Autodesk Inventor part; units mm, degrees
ref_plane "YZ Plane" through (0, 0, 0) normal (1, 0, 0) x (0, 1, 0)
ref_plane "XZ Plane" through (0, 0, 0) normal (0, 1, 0) x (-1, 0, 0)
ref_plane "XY Plane" through (0, 0, 0) normal (0, 0, 1) x (1, 0, 0)
sketch "Esquisse1" plane through (0, 0, 0) normal (0, 0, 1) x (1, 0, 0)
  circle A0 centre (0, 0) radius 13.75
  dimension "d0" = 27.5
extrude "Extrusion1" add sketch "Esquisse1" along normal blind 37.5
sketch "Esquisse2" plane through (0, 0, 0) normal (0, 0, -1) x (-1, 0, 0)
  circle A0 centre (0, 0) radius 5
  dimension "d3" = 10
extrude "Extrusion2" add sketch "Esquisse2" along normal blind 3.5
sketch "Esquisse3" plane through (0, 0, 37.5) normal (0, 0, 1) x (1, 0, 0)
  circle A0 centre (0, 0) radius 1.2
  dimension "d6" = 2.4
extrude "Extrusion3" add sketch "Esquisse3" along normal blind 13
sketch "Esquisse4" plane through (0, 0, 37.5) normal (0, 0, 1) x (1, 0, 0)
  circle A0 centre (0, 0) radius 1.2
  circle A1 centre (0, 0) radius 5
  dimension "d9" = 10
extrude "Extrusion4" add sketch "Esquisse4" along normal blind 3.5
fillet "Congé1" radius 1 2 edges at (-5, 0, 41) (5, 0, -3.5)
fillet "Congé2" radius 1 1 edges at (-13.75, 0, 37.5)
fillet "Congé3" radius 0.5 1 edges at (-1.2, 0, 50.5)
sketch "Esquisse5" plane through (0, 0, 37.5) normal (0, 0, 1) x (1, 0, 0)
  circle A0 centre (0, 8) radius 1
  arc A1 (7.7336, 4.6035) -> (4.9749, 7.5) centre (0, 0) ccw construction
  arc A2 (9.0225, 5.3707) -> (5.8041, 8.75) centre (0, 0) ccw
  arc A3 (6.4446, 3.8362) -> (4.1458, 6.25) centre (0, 0) ccw
  arc A4 (6.4446, 3.8362) -> (9.0225, 5.3707) centre (7.7336, 4.6035) ccw
  arc A5 (5.8041, 8.75) -> (4.1458, 6.25) centre (4.9749, 7.5) ccw
  line L0 (0, 0) -> (0, 21.7918) construction
  circle A6 centre (0, -8) radius 1
  arc A7 (8.75, -5.8041) -> (6.25, -4.1458) centre (7.5, -4.9749) ccw
  arc A8 (5.3707, -9.0225) -> (8.75, -5.8041) centre (0, 0) ccw
  arc A9 (3.8362, -6.4446) -> (5.3707, -9.0225) centre (4.6035, -7.7336) ccw
  arc A10 (3.8362, -6.4446) -> (6.25, -4.1458) centre (0, 0) ccw
  arc A11 (-5.8041, -8.75) -> (-4.1458, -6.25) centre (-4.9749, -7.5) ccw
  arc A12 (-9.0225, -5.3707) -> (-5.8041, -8.75) centre (0, 0) ccw
  arc A13 (-6.4446, -3.8362) -> (-9.0225, -5.3707) centre (-7.7336, -4.6035) ccw
  arc A14 (-6.4446, -3.8362) -> (-4.1458, -6.25) centre (0, 0) ccw
  arc A15 (-8.75, 5.8041) -> (-6.25, 4.1458) centre (-7.5, 4.9749) ccw
  arc A16 (-5.3707, 9.0225) -> (-8.75, 5.8041) centre (0, 0) ccw
  arc A17 (-3.8362, 6.4446) -> (-5.3707, 9.0225) centre (-4.6035, 7.7336) ccw
  arc A18 (-3.8362, 6.4446) -> (-6.25, 4.1458) centre (0, 0) ccw
  dimension "d15" = 2
  dimension "d16" = 3
  dimension "d17" = 8
  dimension "d19" = 7
  dimension "d21" = 5
  dimension "d22" = 9
  dimension "d25" = 360
  dimension "d29" = 360
extrude "Extrusion5" cut sketch "Esquisse5" against normal blind 5
properties part number "Moteur" material "Acier inoxydable"
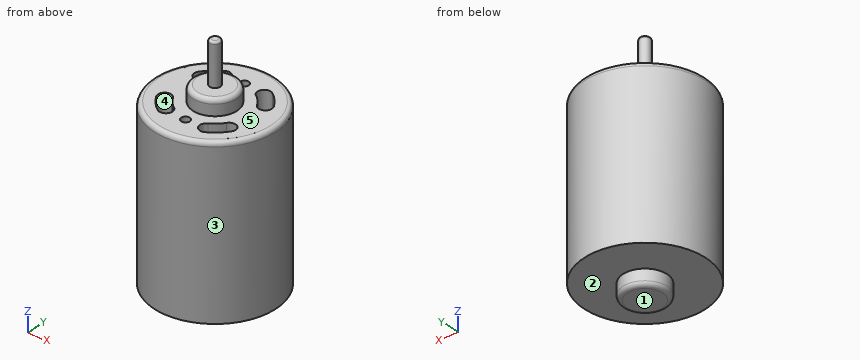
Work out the finished part from the listing and answer in its coordinate system (mm). Face numbers are marked on the shaded views. A direction names the side the tool comes from. Round coordinates to 2 decimals unless told otherwise and drop trailing zeros. Loops run counter-clockwise (first coordinate to the right, second up) from the corner with the lowest first, then second, coordinate; pieces in that order, holes last. Notation, with made-up numbers: (40, 33.5) -> (77, 33.5) arc R18 cw to (77, 67.5) -> close; hole circle Ø8 at (30, -35). An arc over 180 degrees is marked (long way). Write each question's results on one line, items separated by ' | '. Start each with the question number.
1. Find the intervals of material crossed by probe 1 along Y at (x, z) = (0, 34.6); probe 2 along X at (y, z) = (-6, 37); probe 3 along Y at (x, z) = (-0.25, 20.5), in increasing order. Write a range as from..to.
2. A tool of negligible diameter and unlimited length cuts with its end or side. For the marked faces 1 and 2, from which of +Z, -Z, +X, -X, +Y, -Y can it reach the whole face along a straight path? Write none if from no direction.
3. Section D-D (z = 42.5) is taken. Determine the outline of the cut face in (x, y), plus the area to 3 significant figures.
4. Section B-B (y = 0) is taken. Determine the outline of the cut face in (x, z), plus the area to 3 significant figures.
5. Section C-C (z = 28.5) is taken. Determine the outline of the cut face in (x, y), plus the area to 3 significant figures.
6. Given pin 1 Ø1.7 at (x, y) = (7.5, -7) entering from +Z; pin 2 Ø2 at (x, z) = (7.5, 24.5) entering from +Y; pin 3 Ø8 at (y, z) = (6, 30.5) entering from +X, each flat-ended and moving along its own axis, determine where each tip first touches the part or whether it passes through.
7. For a pull along Y with two mould halves and no side action, classify the marked faces 3, 4 and 5 as +Y half, -Y half, draft (parallel to the pull), parting line (faces both ways), or undercut.
Evaluation:
1) probe 1: y = -13.75..-9, -7..7, 9..13.75 | probe 2: x = -12.22..-8.62, -4.5..4.5, 8.62..12.22 | probe 3: y = -13.75..13.75
2) face 1: -Z, +X, -X, +Y, -Y | face 2: -Z
3) outline: circle Ø2.4 at (0, 0) | area: 4.52 mm2
4) outline: (-13.75, 0) -> (-5, 0) -> (-5, -2.5) arc R1 ccw to (-4, -3.5) -> (4, -3.5) arc R1 ccw to (5, -2.5) -> (5, 0) -> (13.75, 0) -> (13.75, 36.5) arc R1 ccw to (12.75, 37.5) -> (5, 37.5) -> (5, 40) arc R1 ccw to (4, 41) -> (1.2, 41) -> (1.2, 50) arc R0.5 ccw to (0.7, 50.5) -> (-0.7, 50.5) arc R0.5 ccw to (-1.2, 50) -> (-1.2, 41) -> (-4, 41) arc R1 ccw to (-5, 40) -> (-5, 37.5) -> (-12.75, 37.5) arc R1 ccw to (-13.75, 36.5) -> close | area: 1,120 mm2
5) outline: circle Ø27.5 at (0, 0) | area: 594 mm2
6) pin 1: stops at z = 37.5 | pin 2: stops at y = 12.12 | pin 3: stops at x = 13.6
7) face 3: parting line | face 4: undercut | face 5: draft
